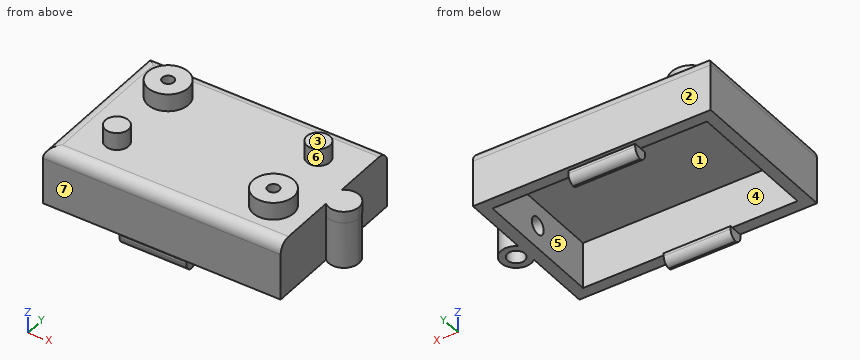
```python
from build123d import *

# Parameters (mm, degrees)
F0_W         = 37
F0_H         = 23
F0_R         = 1.4922705886
F1_DEPTH     = 8
F3_D         = 3
F3_DEPTH     = 4
F3_TIP       = 0.9012909285
F5_DEPTH     = 2
F6_R         = 2
F7_W         = 11.5434788167
F7_H         = 2.4902373552
F8_DEPTH     = 2
F9_T1_DEPTH  = 19.0434788167
F10_T1_DEPTH = 19.0434788167
F11_R        = 3.5
F11_R_2      = 1
F11_R_3      = 2
F12_DEPTH    = 3


# Not quite as in the source:
# - a fillet or chamfer that OpenCascade refuses, or shapes differently, is made with other operations: its cross-section is extruded or revolved along the edge and cut away or added


with BuildPart() as f1:
    # F0 (on Top) → F1 (new body)
    with BuildSketch(Plane.XY):
        with BuildLine():
            Line((-10.4036603272, 27), (-51.4036603272, 27))
            Line((-51.4036603272, 27), (-51.4036603272, 0))
            Line((-51.4036603272, 0), (-10.4036603272, 0))
            Line((-10.4036603272, 0), (-10.4036603272, 11.5282175104))
            ThreePointArc((-10.4036603272, 11.5282175104), (-11.2988558778, 13.5), (-10.4036603272, 15.4717824896))
            Line((-10.4036603272, 15.4717824896), (-10.4036603272, 27))
        make_face()
        with Locations((-30.9036603272, 13.5)):
            Rectangle(F0_W, F0_H, mode=Mode.SUBTRACT)
        with BuildLine():
            ThreePointArc((-6.0605576566, 13.5), (-7.5969670408, 15.8848724805), (-10.4036603272, 15.4717824896))
            Line((-10.4036603272, 15.4717824896), (-10.4036603272, 11.5282175104))
            ThreePointArc((-10.4036603272, 11.5282175104), (-7.5969670408, 11.1151275195), (-6.0605576566, 13.5))
        make_face()
        with Locations((-8.6797067672, 13.5)):
            Circle(F0_R, mode=Mode.SUBTRACT)
        with BuildLine():
            Line((-10.4036603272, 11.5282175104), (-10.4036603272, 15.4717824896))
            ThreePointArc((-10.4036603272, 15.4717824896), (-11.2988558778, 13.5), (-10.4036603272, 11.5282175104))
        make_face()
    extrude(amount=F1_DEPTH)

    # F3 (one way)
    with BuildSketch(Plane(origin=(-12.4036603272, 0, 0), x_dir=(0, -1, 0), z_dir=(-1, 0, 0))):
        with Locations((-13.5, 4)):
            Circle(F3_D / 2)
    extrude(amount=-F3_DEPTH, mode=Mode.SUBTRACT)
    with Locations(Plane(origin=(-12.4036603272, 0, 0), x_dir=(0, -1, 0), z_dir=(-1, 0, 0))):
        with Locations((-13.5, 4)):
            with Locations((0, 0, -(F3_DEPTH + F3_TIP / 2))):  # 118° drill point
                Cone(0, F3_D / 2, F3_TIP, mode=Mode.SUBTRACT)

    # F4 (on face) → F5 (join)
    with BuildSketch(Plane.XY.offset(8)):
        with BuildLine():
            Line((-10.4036603272, 27), (-51.4036603272, 27))
            Line((-51.4036603272, 27), (-51.4036603272, 0))
            Line((-51.4036603272, 0), (-10.4036603272, 0))
            Line((-10.4036603272, 0), (-10.4036603272, 11.4980807802))
            ThreePointArc((-10.4036603272, 11.4980807802), (-11.3216182797, 13.5), (-10.4036603272, 15.5019192198))
            Line((-10.4036603272, 15.5019192198), (-10.4036603272, 27))
        make_face()
        with BuildLine():
            ThreePointArc((-6.0377952547, 13.5), (-7.5785338283, 15.9014817506), (-10.4036603272, 15.5019192198))
            Line((-10.4036603272, 15.5019192198), (-10.4036603272, 11.4980807802))
            ThreePointArc((-10.4036603272, 11.4980807802), (-7.5785338283, 11.0985182494), (-6.0377952547, 13.5))
        make_face()
        with BuildLine():
            Line((-10.4036603272, 11.4980807802), (-10.4036603272, 15.5019192198))
            ThreePointArc((-10.4036603272, 15.5019192198), (-11.3216182797, 13.5), (-10.4036603272, 11.4980807802))
        make_face()
    extrude(amount=F5_DEPTH)

    # F6
    f6_edges = [f1.edges().sort_by_distance(p)[0] for p in [
        (-51.40366, 13.5, 10),
        (-30.90366, 27, 10),
        (-30.90366, 0, 10),
    ]]
    fillet(f6_edges, radius=F6_R)

    # F7 (on Top) → F8 (join)
    with BuildSketch(Plane.XY):
        with Locations((-32.3717817664, 1.1760484776)):
            Rectangle(F7_W, F7_H)
        with Locations((-32.1847852319, 25.1162685454)):
            Rectangle(F7_W, F7_H)
    extrude(amount=-F8_DEPTH)

    # F9: fillet of radius 1.5 on 2 edges, made by hand

    # F9_s2 → F9_t1 (cut)
    with BuildSketch(Plane.YZ.offset(-41.7065246403)):
        with BuildLine():
            ThreePointArc((26.361387223, -0.5), (25.9220473948, -1.5606601718), (24.861387223, -2))
            Line((24.861387223, -2), (26.361387223, -2))
            Line((26.361387223, -2), (26.361387223, -0.5))
        make_face()
        with BuildLine():
            ThreePointArc((23.8711498678, -0.5), (24.310489696, -1.5606601718), (25.3711498678, -2))
            Line((25.3711498678, -2), (23.8711498678, -2))
            Line((23.8711498678, -2), (23.8711498678, -0.5))
        make_face()
    extrude(amount=F9_T1_DEPTH, mode=Mode.SUBTRACT)

    # F10: fillet of radius 1.5 on 2 edges, made by hand

    # F10_s2 → F10_t1 (cut)
    with BuildSketch(Plane.YZ.offset(-41.8935211748)):
        with BuildLine():
            ThreePointArc((2.4211671553, -0.5), (1.981827327, -1.5606601718), (0.9211671553, -2))
            Line((0.9211671553, -2), (2.4211671553, -2))
            Line((2.4211671553, -2), (2.4211671553, -0.5))
        make_face()
        with BuildLine():
            ThreePointArc((-0.0690702, -0.5), (0.3702696283, -1.5606601718), (1.4309298, -2))
            Line((1.4309298, -2), (-0.0690702, -2))
            Line((-0.0690702, -2), (-0.0690702, -0.5))
        make_face()
    extrude(amount=F10_T1_DEPTH, mode=Mode.SUBTRACT)

    # F11 (on face) → F12 (join)
    with BuildSketch(Plane.XY.offset(10)):
        with Locations((-16.4036603272, 7)):
            Circle(F11_R)
        with Locations((-16.4036603272, 7)):
            Circle(F11_R_2, mode=Mode.SUBTRACT)
        with Locations((-43.4036603272, 7)):
            Circle(F11_R_3)
        with Locations((-43.4036603272, 20)):
            Circle(F11_R)
        with Locations((-43.4036603272, 20)):
            Circle(F11_R_2, mode=Mode.SUBTRACT)
        with Locations((-17.4769777805, 20)):
            Circle(F11_R_3)
    extrude(amount=F12_DEPTH)


solid = f1.part
```
Could you check a few things on this model? Use its own coordinates, in mm. Face numbers are marked on the shaded views. A direction names the side the tool comes from. Round coordinates to 2 decimals unless told otherwise and drop trailing zeros. Loops run counter-clockwise (first coordinate to the right, second up) from the corner with the lowest first, then second, coordinate; pieces in that order, holes last. Notation, with made-up numbers: M -35,54.5 L 16,54.5 A18 cw 16,77.5 Z; hole C 37.5,72 d7. An arc over 180 degrees is marked long. Put each result on its own line as item: value.
Q1. For pin 1 (4 mm diameter, centred on x = -25, z = 7.5, fed in from -Y); pin 2 (2 mm diameter, centred on x = -16.5, y = 7, fed in from +Z); pin 3 (0.5 mm diameter, centred on x = -30, y = 2, fed in from +Z); pin 4 (1.6 mm diameter, centred on x = -43.4, y = 20, fed in from -Z), each with a flat end and sliding along its axis, tell me the tip position at first contact or that it passes through.
Check result:
pin 1: y = 0
pin 2: z = 13
pin 3: z = 10
pin 4: z = 8
Q2. Thinking about a two-plate mould opening in Y: for the marked faces 1, 2 and 3, which applies, released by +Y, released by -Y, zero draft, split by the parting line, or undercut?
Check result:
face 1: undercut
face 2: released by +Y
face 3: zero draft
Q3. Imagine slicing it at D-D (z = 6.75). Write out the boundary of the cut face in (x, y), then the cut area to 3 significant figures.
Check result:
outline: M -51.4,0 L -10.4,0 L -10.4,11.53 A2.62 ccw long -10.4,15.47 L -10.4,27 L -51.4,27 Z; hole M -49.4,2 L -12.4,2 L -12.4,25 L -49.4,25 Z; hole C -8.68,13.5 d2.98
area: 268 mm2
Q4. Imagine slicing it at A-A (z = 11.75). Write out the boundary of the cut face in (x, y).
Check result:
outline: C -43.4,20 d7; C -43.4,7 d4; C -16.4,7 d7; C -17.48,20 d4; hole C -43.4,20 d2; hole C -16.4,7 d2
Q5. On a 3-axis mill with a long thin cutter (end or side, diameter ignored), from which of +Z, -Z, +X, -X, +Y, -Y can I reach the whole of each face in a straight line? I mean the marked faces 4, 5, 6 and 7. Say none if no direction works.
Check result:
face 4: none
face 5: -Z
face 6: +Z
face 7: +Z, +X, -X, -Y
Q6. Imagine slicing it at B-B (x = -32.5). Write out the boundary of the cut face in (y, z).
Check result:
outline: M -0.07,-0.5 A1.5 ccw 1.18,-1.98 A1.5 ccw 2.42,-0.5 L 2.42,0 L 2,0 L 2,8 L 25,8 L 25,0 L 23.87,0 L 23.87,-0.5 A1.5 ccw 25.12,-1.98 A1.5 ccw 26.36,-0.5 L 26.36,0 L 27,0 L 27,8 A2 ccw 25,10 L 2,10 A2 ccw 0,8 L 0,0 L -0.07,0 Z
Q7. Imagine slicing it at C-C (y = 7). Write out the boundary of the cut face in (x, z).
Check result:
outline: M -51.4,0 L -49.4,0 L -49.4,8 L -12.4,8 L -12.4,0 L -10.4,0 L -10.4,10 L -12.9,10 L -12.9,13 L -15.4,13 L -15.4,10 L -17.4,10 L -17.4,13 L -19.9,13 L -19.9,10 L -41.4,10 L -41.4,13 L -45.4,13 L -45.4,10 L -49.4,10 A2 ccw -51.4,8 Z
Q8. I need wall thicknesses on probe 1 along Y at (x, z) = (-42.5, 6.5); probe 2 along X at (y, z) = (13.5, 5.25); probe 3 along X at (y, z) = (23.25, 0.75). Which ranges of each line are inside material? Lowest first, please.
Check result:
probe 1: 0 to 2, 25 to 27
probe 2: -51.4 to -49.4, -7.19 to -6.06
probe 3: -51.4 to -49.4, -12.4 to -10.4
